```python
from build123d import *

# Parameters (mm, degrees)
EXTRUDE_1_DEPTH     = 40
SKETCH_2_R          = 2.75
CUT_EXTRUDE_1_DEPTH = 40


with BuildPart() as part:
    # 草图1 → 凸台-拉伸1 (new body)
    with BuildSketch(Plane.XY):
        Polygon((0, 0), (0, -2), (40, -2), (40, 38), (38, 38), (38, 0), align=None)
    extrude(amount=EXTRUDE_1_DEPTH)

    # 草图2 → 切除-拉伸1 (cut)
    with BuildSketch(Plane(origin=(40, 0, 0), x_dir=(0, 0, -1), z_dir=(1, 0, 0))):
        with Locations((-30, 31)):
            Circle(SKETCH_2_R)
        with Locations(Location((-10, 31, 0), (0, 0, 90))):
            Circle(SKETCH_2_R)
    cut_extrude_1 = extrude(amount=-CUT_EXTRUDE_1_DEPTH, mode=Mode.SUBTRACT)

    # 镜向1: 切除-拉伸1 across plane
    add(cut_extrude_1.mirror(Plane(origin=(19, 19, 0), x_dir=(0, 0, 1), z_dir=(0.7071067811865488, 0.7071067811865464, 0))), mode=Mode.SUBTRACT)


solid = part.part
```
The listing builds one solid part. Answer for the finished solid, in the listing's coordinates (mm). A direction names the side the tool comes from. Give positions to 0.01 mm unless a question says otherwise; leave off trailing zeros. Write each loop counter-clockwise with the first axis right and the second up, starting at its lowest first coordinate (ties: lowest second). Pieces come first, ordered by that corner, then holes. Notation, with made-up numbers: (14, 23.5) -> (19, 23.5) arc R26 ccw to (19, 41.5) -> close; hole circle Ø5 at (40.5, -39.5). An arc over 180 degrees is marked (long way). Use one line per item in the form item = value.
1) A tool of negligible diameter and unlimited length cuts with its end or side. For faces 1 (the flat face through (0, -1, 20)), 2 (the flat face through (38, 19, 20)), from which of +Z, -Z, +X, -X, +Y, -Y can it reach the whole face along a straight path? Write none if from no direction.
Result:
face_1 = +Z, -Z, -X, +Y, -Y
face_2 = +Z, -Z, -X, +Y
2) Section B-B on y = 31 is taken. Write down the section's boundary in (x, z), plus the area to 3 significant figures.
Result:
outline = (38, 0) -> (40, 0) -> (40, 7.25) -> (38, 7.25) -> close; (38, 12.75) -> (40, 12.75) -> (40, 27.25) -> (38, 27.25) -> close; (38, 32.75) -> (40, 32.75) -> (40, 40) -> (38, 40) -> close
area = 58.0 mm²
3) Section A-A on z = 30 is taken. Write down the section's boundary in (x, y), plus the area to 3 significant figures.
Result:
outline = (0, -2) -> (4.25, -2) -> (4.25, 0) -> (0, 0) -> close; (9.75, -2) -> (40, -2) -> (40, 28.25) -> (38, 28.25) -> (38, 0) -> (9.75, 0) -> close; (38, 33.75) -> (40, 33.75) -> (40, 38) -> (38, 38) -> close
area = 134 mm²
4) For a pull along Y with two mould halves and no side action, classify faces 3 (the flat face through (19, 0, 20)), 4 (the flat face through (29, -1, 0)), 5 (the cylindrical face through (39.014, 28.253, 10.121)) as +Y half, -Y half, draft (parallel to the pull), parting line (faces both ways), or undercut.
Result:
face_3 = +Y half
face_4 = draft
face_5 = undercut
5) Section D-D on z = 20 is taken. Write down the section's boundary in (x, y).
Result:
outline = (0, -2) -> (40, -2) -> (40, 38) -> (38, 38) -> (38, 0) -> (0, 0) -> close
6) Section C-C on x = 5 is taken. Write down the section's boundary in (y, z).
Result:
outline = (-2, 0) -> (0, 0) -> (0, 8.11) -> (-2, 8.11) -> close; (-2, 11.89) -> (0, 11.89) -> (0, 28.11) -> (-2, 28.11) -> close; (-2, 31.89) -> (0, 31.89) -> (0, 40) -> (-2, 40) -> close
7) Each of these flat-tipped pins is pushed along its axis until it touches: P1, Ø6.5, axis at y = 31, z = 30, coming from the -X side; P2, Ø7, axis at x = 7, z = 10, coming from the -Y side; P3, Ø1.5, axis at x = 26, z = 21, coming from the +Y side. Where does it stop, or does it pass through?
Result:
P1 = 38
P2 = -2
P3 = 0
8) Straight lines are drawn through the part: probe 1 along Z at (x, y) = (7, -1.35); probe 2 along Y at (x, z) = (38.95, 30); probe 3 along X at (y, z) = (-1, 10). For each, find the intervals that lie inside material, in ascending order.
Result:
probe_1 = 0 to 7.25, 12.75 to 27.25, 32.75 to 40
probe_2 = -2 to 28.25, 33.75 to 38
probe_3 = 0 to 4.25, 9.75 to 40
